Autodesk Inventor part; units mm, degrees
ref_plane "YZ Plane" through (0, 0, 0) normal (1, 0, 0) x (0, 1, 0)
ref_plane "XZ Plane" through (0, 0, 0) normal (0, 1, 0) x (-1, 0, 0)
ref_plane "XY Plane" through (0, 0, 0) normal (0, 0, 1) x (1, 0, 0)
sketch "スケッチ1" plane through (0, 0, 0) normal (0, 1, 0) x (-1, 0, 0)
  circle A0 centre (0, 0) radius 1.075
  line L0 (-2.5, -2.5) -> (2.5, -2.5)
  line L1 (2.5, -2.5) -> (2.5, 2.5)
  line L2 (2.5, 2.5) -> (-2.5, 2.5)
  line L3 (-2.5, 2.5) -> (-2.5, -2.5)
  line L4 (-2.5, -2.5) -> (2.5, 2.5) construction
  line L5 (2.5, -2.5) -> (-2.5, 2.5) construction
  dimension "d0" = 2.15
  dimension "d1" = 5
  dimension "d2" = 5
extrude "押し出し1" add sketch "スケッチ1" along normal blind 100 contours A0 | L3 L2 L1 L0
extrude "押し出し2" cut sketch "スケッチ1" along normal blind 15 contours A0
sketch "スケッチ2" plane through (0, 100, 0) normal (0, 1, 0) x (1, 0, 0)
  point P0 (0, 0)
hole "穴1" at (0, 100, 0) direction (0, -1, 0) diameter 2.15 depth 50 tip angle 118
sketch "スケッチ3" plane through (2.5, 0, -2.5) normal (0, 0, -1) x (-1, 0, 0)
  line L0 (5, 0) -> (0, 0)
  line L1 (5, 0) -> (5, 100)
  line L2 (0, 0) -> (5, 0)
  line L3 (5, 0) -> (5, 15)
  line L4 (5, 15) -> (0, 15)
  line L5 (0, 15) -> (0, 0)
  circle A0 centre (2.5, 15) radius 1
  line L6 (0, 100) -> (5, 100)
  line L7 (0, 100) -> (5, 100)
  line L8 (5, 100) -> (5, 50)
  line L9 (5, 50) -> (0, 50)
  line L10 (0, 50) -> (0, 100)
  circle A1 centre (2.5, 50) radius 1.1
  point P0 (2.5, 0)
  dimension "d14" = 15
  dimension "d15" = 2
  dimension "d16" = 50
  dimension "d17" = 2.2
extrude "押し出し3" cut sketch "スケッチ3" against normal blind 5 contours A0 L4 | L4 A0 | A1 L9 | L9 A1
properties part number "g_a_exp"
CAD build for the part. Positions are in the model's coordinates, mm. A direction names the side the tool comes from. Give positions to 0.01 mm unless a question says otherwise; leave off trailing zeros. Write each loop counter-clockwise with the first axis right and the second up, starting at its lowest first coordinate (ties: lowest second). Pieces come first, ordered by that corner, then holes. Notation, with made-up numbers: M -2,75.5 L 43,75.5 A16 cw 43,84.5 Z; hole C 32,-38 d6. An arc over 180 degrees is marked long. Put each result on its own line as item: value. Start each with the question number.
(1) Probe L1, parallel to X at y = 15, z = -1.05; L2, parallel to X at y = 50, z = 0.7. List the from-to ranges inside material, lowest first.
(2) Which spindle directions (+Z, -Z, +X, -X, +Y, -Y) get a long thin tool onto all of the face, cutting with end or side? Do faces 1 (the face through (2.5, 49, 0)), 2 (the face through (-1.025, 7.395, -0.323)). Say none if no direction does.
(3) Band-saw the part on A-A, the plane y = 85. Write the cut outline in (x, z) (3 decimals), and give its area (3 significant figures).
(4) Flat gauge pins, fed straight in: pin 1 Ø3 at (x, y) = (0, 50) entering from +Z; pin 2 Ø1.3 at (x, z) = (0, 0) entering from +Y. Where does each tip first touch, or does it go through?
(5) Mould opens along Z. For faces 3 (the face through (-1, 49, -2.5)), 4 (the face through (-0.323, 74.768, 1.025)), 5 (the face through (1, 49, 2.5)), 6 (the face through (-2.5, 49, 0)) say: +Z half, -Z half, draft (parallel to the pull), parting line (faces both ways), or undercut.
Response values:
1. L1: x = -2.5 to -1, 1 to 2.5
1. L2: x = -2.5 to -1.1, 1.1 to 2.5
2. face 1: +Z, -Z, +X, +Y, -Y
2. face 2: -Y
3. outline: M -2.5,-2.5 L 2.5,-2.5 L 2.5,2.5 L -2.5,2.5 Z; hole C 0,0 d2.15
3. area: 21.4 mm2
4. pin 1: stops at z = 2.5
4. pin 2: stops at y = 49.11
5. face 3: -Z half
5. face 4: undercut
5. face 5: +Z half
5. face 6: draft
